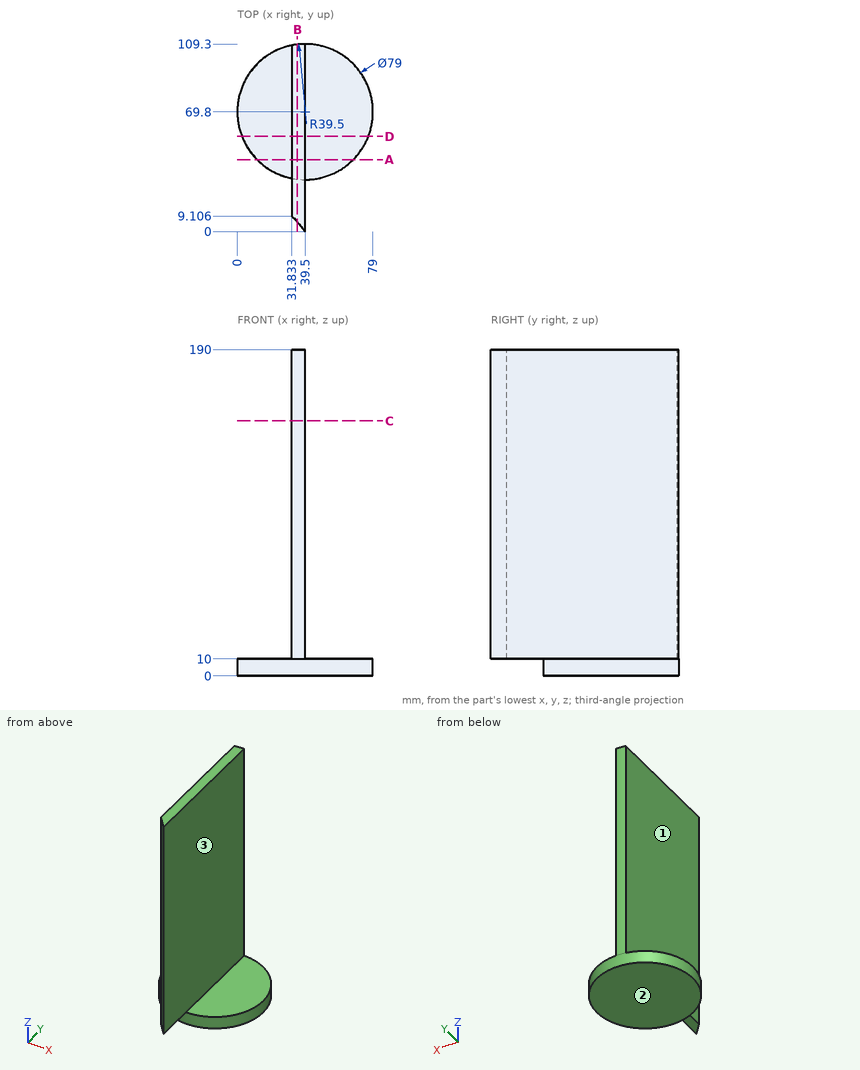
The drawing under review shows one solid part. Ordinate dimensions are in mm from its lowest x, y, z. A direction names the side the tool comes from. Give positions to 0.01 mm unless a question says otherwise; leave off trailing zeros. Write each loop counter-clockwise with the first axis right and the second up, starting at its lowest first coordinate (ties: lowest second). Pieces come first, ordered by that corner, then holes. Notation, with made-up numbers: (-27, 70.5) - (-4, 70.5) arc R33 ccw to (-4, 109.5) - close; hole circle Ø6 at (41, 19). An arc over 180 degrees is marked (long way). Answer in a Markdown table with one row per item. Add a question column.
1. Tool access review of the marked faces 1, 2 and 3: name each direction out of +Z, -Z, +X, -X, +Y, -Y from which nothing blocks a thin tool from reaching the whole face with its end or side.
2. We need section A-A on y = 42. Write out the cut boundary in (x, z).
3. We need section B-B on x = 35. Write out the cut boundary in (y, z), then the cut area to 3 significant figures.
4. Insertion check: P1, Ø6, axis at x = 15, y = 85, coming from the +Z side; P2, Ø2.5, axis at x = 36, y = 16, coming from the -Z side; P3, Ø10, axis at y = 58, z = 96, coming from the +X side. Each pin has a flat end and moves straight along its axis. Give the tip position at first contact, or say it passes through.
5. We need section C-C on z = 148.5. Write out the cut boundary in (x, y), then the cut area to 3 significant figures.
6. We need section D-D on y = 55.5. Write out the cut boundary in (x, z), then the cut area to 3 significant figures.
7. Wall thickness on line 1 along Z through (x, y) = (46.5, 69.5); line 2 along X through (y, z) = (97.5, 160.5); line 3 along Y through (x, z) = (26, 9.5): over which ranges is each line inside the solid? List them lowest first. Write a range as [from, to].
Ans:
| question | item | result |
|---|---|---|
| 1 | face 1 | +Z, -X, +Y, -Y |
| 1 | face 2 | -Z, +X, -X, +Y, -Y |
| 1 | face 3 | +Z, +X, +Y, -Y |
| 2 | outline | (11.44, 0) - (67.56, 0) - (67.56, 10) - (39.5, 10) - (39.5, 190) - (31.83, 190) - (31.83, 10) - (11.44, 10) - close |
| 3 | outline | (5.34, 10) - (30.56, 10) - (30.56, 0) - (109.04, 0) - (109.04, 190) - (5.34, 190) - close |
| 3 | area | 19,500 mm^2 |
| 4 | P1 | stops at z = 10 |
| 4 | P2 | stops at z = 10 |
| 4 | P3 | stops at x = 39.5 |
| 5 | outline | (31.83, 9.11) - (39.5, 0) - (39.5, 109.3) arc R39.5 ccw to (31.83, 108.55) - close |
| 5 | area | 801 mm^2 |
| 6 | outline | (2.68, 0) - (76.32, 0) - (76.32, 10) - (39.5, 10) - (39.5, 190) - (31.83, 190) - (31.83, 10) - (2.68, 10) - close |
| 6 | area | 2,120 mm^2 |
| 7 | line 1 | z = [0, 10] |
| 7 | line 2 | x = [31.83, 39.5] |
| 7 | line 3 | y = [32.68, 106.92] |
